For this review, take the finished solid that the model builds, in its own axes (mm). Face numbers are marked on the shaded views. Round coordinates to 2 decimals unless told otherwise and drop trailing zeros. Order: outer loops, then holes, each group sorted by start corner. A loop starts at its lowest first (then second) coordinate and runs counter-clockwise, first axis right, second up. Notation, with made-up numbers: M 68.5,55 L 125.5,55 A28 cw 125.5,92 Z; hole C 70,86.5 d1. An arc over 180 degrees is marked long. Put each result on its own line as item: value.
from build123d import *

# Parameters (mm, degrees)
F1_DEPTH = 6
F2_DEPTH = 3


with BuildPart() as f1:
    # F0 (on Top) → F1 (new body)
    with BuildSketch(Plane.XY):
        with BuildLine():
            Line((-44.7939935698, 3.25), (-5.1229558211, 3.25))
            ThreePointArc((-5.1229558211, 3.25), (-6.0793955706, 0), (-5.1229558211, -3.25))
            Line((-5.1229558211, -3.25), (-44.7939935698, -3.25))
            ThreePointArc((-44.7939935698, -3.25), (-42.6572806733, -5.2490864776), (-39.8292040073, -6))
            Line((-39.8292040073, -6), (-0.0793955706, -6))
            ThreePointArc((-0.0793955706, -6), (5.9206044294, 0), (-0.0793955706, 6))
            Line((-0.0793955706, 6), (-39.8292040073, 6))
            ThreePointArc((-39.8292040073, 6), (-42.6572806733, 5.2490864776), (-44.7939935698, 3.25))
        make_face()
        with BuildLine():
            ThreePointArc((-1.6613247726, 2), (1.0315905983, 2.2952580971), (2.4706044294, 0))
            ThreePointArc((2.4706044294, 0), (1.0315905983, -2.2952580971), (-1.6613247726, -2))
            ThreePointArc((-1.6613247726, -2), (-2.6293955706, 0), (-1.6613247726, 2))
        make_face(mode=Mode.SUBTRACT)
        with BuildLine():
            Line((-1.6613247726, -2), (-1.6613247726, 2))
            ThreePointArc((-1.6613247726, 2), (-2.6293955706, 0), (-1.6613247726, -2))
        make_face()
    extrude(amount=F1_DEPTH)

    # F0 (on Top) → F2 (join)
    with BuildSketch(Plane.XY):
        with BuildLine():
            ThreePointArc((-5.1229558211, -3.25), (-6.0793955706, 0), (-5.1229558211, 3.25))
            Line((-5.1229558211, 3.25), (-44.7939935698, 3.25))
            ThreePointArc((-44.7939935698, 3.25), (-45.7503337184, 0), (-44.7939935698, -3.25))
            Line((-44.7939935698, -3.25), (-5.1229558211, -3.25))
        make_face()
    extrude(amount=F2_DEPTH)


solid = f1.part
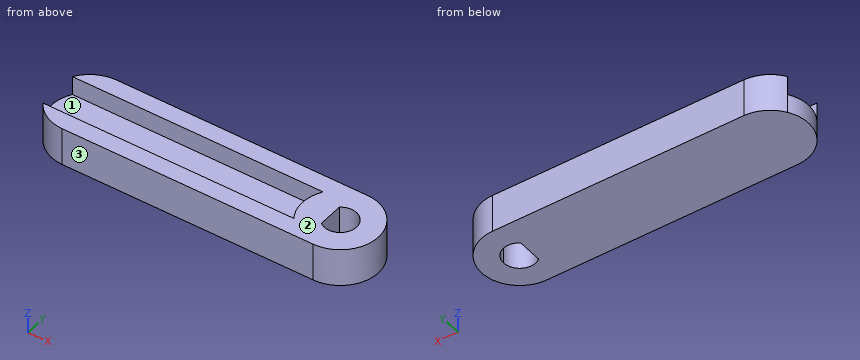
(1) Add section B-B on x = -35.5. Give the boundary of the cut face in (y, z), then the cut area to 3 significant figures.
A:
outline: M -6,0 L 6,0 L 6,6 L 3.25,6 L 3.25,3 L -3.25,3 L -3.25,6 L -6,6 Z
area: 52.5 mm2
(2) Add section D-D on x = 0.5. Give the boundary of the cut face in (y, z), then the cut area to 3 significant figures.
A:
outline: M -5.97,0 L -2.48,0 L -2.48,6 L -5.97,6 Z; M 2.48,0 L 5.97,0 L 5.97,6 L 2.48,6 Z
area: 41.9 mm2
(3) Insertion check: pin 1 Ø1.2 at (y, z) = (-1, 3.5) entering from +X; pin 2 Ø4 at (x, y) = (-16, -1.5) entering from -Z; pin 3 Ø2 at (x, y) = (-29.5, 1) entering from +Z; pin 4 Ø3 at (y, z) = (2.5, 5) entering from -X. Each pin has a flat end and moves straight along its axis. Give the tip position at first contact, or say it passes through.
A:
pin 1: stops at x = 5.91
pin 2: stops at z = 0
pin 3: stops at z = 3
pin 4: stops at x = -44.79
(4) Add section A-A on z = 3.5. Give the boundary of the cut face in (x, y), then the cut area to 3 significant figures.
A:
outline: M -44.79,-3.25 A6 ccw -39.83,-6 L -0.08,-6 A6 ccw -0.08,6 L -39.83,6 A6 ccw -44.79,3.25 L -5.12,3.25 A6 ccw -5.12,-3.25 Z; hole M -1.66,-2 A2.55 ccw long -1.66,2 Z
area: 314 mm2
(5) Add section C-C on y = 1.25. Give the boundary of the cut face in (x, z).
A:
outline: M -45.62,0 L -1.66,0 L -1.66,6 L -5.95,6 L -5.95,3 L -45.62,3 Z; M 2.14,0 L 5.79,0 L 5.79,6 L 2.14,6 Z
(6) To check wall thickness, follow L1, parallel to Y at x = -18, z = 5.2; L2, parallel to Z at x = -26.5, y = 0.5. State the ranges of each line that lie inside material, in increasing order.
A:
L1: y = -6 to -3.25, 3.25 to 6
L2: z = 0 to 3
(7) Draft analysis for pull direction Y (two halves, no side actions). For the marked faces 1, 2 and 3, state which applies: released by +Y, released by -Y, zero draft, split by the parting line, or undercut.
A:
face 1: undercut
face 2: zero draft
face 3: released by -Y
